Can you work these out from the drawing? Everything is in mm from the part's minimum corner. A direction names the side the tool comes from. Give positions to 0.01 mm unless a question says otherwise; leave off trailing zeros. Write each loop counter-clockwise with the first axis right and the second up, starting at its lowest first coordinate (ties: lowest second). Pieces come first, ordered by that corner, then holes. Notation, with made-up numbers: (56, 75) - (115, 75) arc R31 ccw to (115, 108) - close; hole circle Ø5 at (-27.5, 78). An arc over 180 degrees is marked (long way). Return JSON: item names as keys, results as strings. Group by question number.
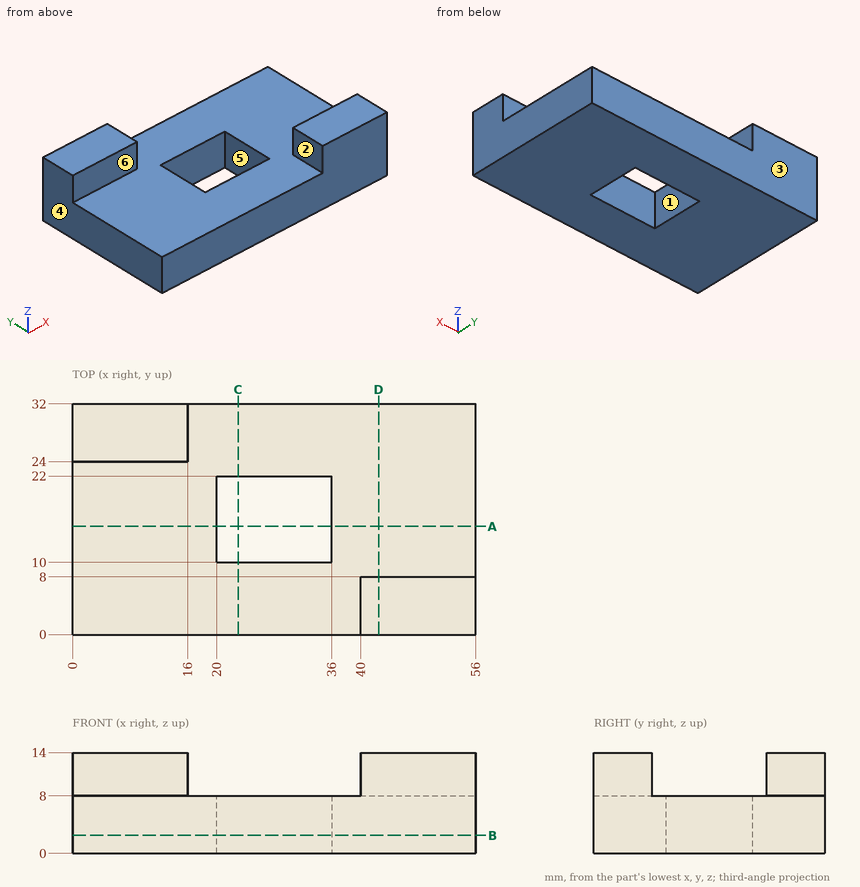
1) Imagine slicing it at D-D, the plane x = 42.5. Write out the boundary of the cut face in (y, z).
2) Imagine slicing it at C-C, the plane x = 23. Write out the boundary of the cut face in (y, z).
3) We'd pull the mould along Y, two halves only. Please class the marked faces 1, 2 and 3: pulls with the +Y half, pulls with the -Y half, needs draft (parallel to the pull), parting line crosses it, or undercut.
4) On a 3-axis mill with a long thin cutter (end or side, diameter ignored), from which of +Z, -Z, +X, -X, +Y, -Y can I reach the whole of each face in a straight line? I mean the marked faces 4, 5 and 6. Say none if no direction works.
5) Imagine slicing it at B-B, the plane z = 2.5. Write out the boundary of the cut face in (x, y), and give its area (3 significant figures).
6) Will these pins go through, and if not, where does the flat tip stop? pin 1 Ø16 at (x, y) = (15, 22.5) entering from +Z; pin 2 Ø6.5 at (x, z) = (6.5, 12.5) entering from -Y; pin 3 Ø3 at (y, z) = (29.5, 11) entering from +X; pin 4 Ø5 at (y, z) = (20.5, 12) entering from +X.
7) Imagine slicing it at A-A, the plane y = 15. Write out the boundary of the cut face in (x, z), and give its area (3 significant figures).
8) I need wall thicknesses on line 1 along X through (y, z) = (11, 6.5); line 2 along Y through (x, z) = (24.5, 6.75); line 3 along X through (y, z) = (7.5, 12.75). Which ranges of each line are inside material? Lowest first, please.
Resolved:
{
 "1": {"outline": "(0, 0) - (32, 0) - (32, 8) - (8, 8) - (8, 14) - (0, 14) - close"},
 "2": {"outline": "(0, 0) - (10, 0) - (10, 8) - (0, 8) - close; (22, 0) - (32, 0) - (32, 8) - (22, 8) - close"},
 "3": {"face 1": "undercut", "face 2": "needs draft", "face 3": "pulls with the +Y half"},
 "4": {"face 4": "+Z, -Z, -X, +Y, -Y", "face 5": "+Z, -Z", "face 6": "+Z, +X, -X, -Y"},
 "5": {"outline": "(0, 0) - (56, 0) - (56, 32) - (0, 32) - close; hole (20, 10) - (36, 10) - (36, 22) - (20, 22) - close", "area": "1,600 mm^2"},
 "6": {"pin 1": "z = 14", "pin 2": "y = 24", "pin 3": "x = 16", "pin 4": "through"},
 "7": {"outline": "(0, 0) - (20, 0) - (20, 8) - (0, 8) - close; (36, 0) - (56, 0) - (56, 8) - (36, 8) - close", "area": "320 mm^2"},
 "8": {"line 1": "0 to 20, 36 to 56", "line 2": "0 to 10, 22 to 32", "line 3": "40 to 56"}
}
